```python
from build123d import *

# Parameters (mm, degrees)
F1_DEPTH = 38.1
F2_DEPTH = 63.5
F3_R     = 12.703802
F4_DEPTH = 65.251941


with BuildPart() as f1:
    # F0 (on Front) → F1 (new body, symmetric)
    with BuildSketch(Plane.XZ):
        with BuildLine():
            Line((-25.716836, 32.62547), (-67.867137, 32.62547))
            Line((-67.867137, 32.62547), (-67.867137, -32.62547))
            Line((-67.867137, -32.62547), (67.867137, -32.62547))
            Line((67.867137, -32.62547), (67.867137, 32.62547))
            Line((67.867137, 32.62547), (25.716836, 32.62547))
            ThreePointArc((25.716836, 32.62547), (0, 6.908634), (-25.716836, 32.62547))
        make_face()
    extrude(amount=F1_DEPTH, both=True)

    # F0 (on Front) → F2 (join, symmetric)
    with BuildSketch(Plane.XZ):
        with BuildLine():
            Line((-15.157554, 32.62547), (-25.716836, 32.62547))
            ThreePointArc((-25.716836, 32.62547), (0, 6.908634), (25.716836, 32.62547))
            Line((25.716836, 32.62547), (15.157554, 32.62547))
            ThreePointArc((15.157554, 32.62547), (0, 17.467917), (-15.157554, 32.62547))
        make_face()
    extrude(amount=F2_DEPTH, both=True)

    # F3 (on face) → F4 (cut, through all)
    with BuildSketch(Plane.XY.offset(32.62547)):
        with Locations((-43.029986, 0)):
            Circle(F3_R)
        with Locations((43.029986, 0)):
            Circle(F3_R)
    extrude(amount=-F4_DEPTH, mode=Mode.SUBTRACT)


solid = f1.part
```
Geometry check sheet. Reference: the model listing, model coordinates, mm. A direction names the side the tool comes from. Coordinates: 2 decimals unless noted, no trailing zeros. Write each loop counter-clockwise with the first axis right and the second up, starting at its lowest first coordinate (ties: lowest second). Pieces come first, ordered by that corner, then holes. Notation, with made-up numbers: (34.5, -22.5) -> (76.5, -22.5) arc R20 cw to (76.5, 2.5) -> close; hole circle Ø6 at (34.25, 51). An arc over 180 degrees is marked (long way). Use CSV: the item, a comma, the result in double quotes. Start each with the question number.
Item 1: Cross-section at D-D, the plane z = 14. Record the cut outline in (x, y).
Item 2: Mould release check, pull along X, two halves, no side actions. Record for faces 1 (the cylindrical face through (30.34, 0.56, 0.46)), 2 (the flat face through (-67.867, -1, 0)), 3 (the flat face through (0, 63.5, 17)), 4 (the flat face through (67.867, -1, 0)): released by +X, released by -X, zero draft, split by the parting line, or undercut.
Item 3: Cross-section at C-C, the plane y = 0. Record the cut outline in (x, z).
Item 4: Set-up check for faces 5 (the flat face through (30, -1, 32.625)), 6 (the cylindrical face through (-0.565, -50.978, 6.915)), 7 (the flat face through (-1, 38.1, 0)): record each of +Z, -Z, +X, -X, +Y, -Y from which the full face is reachable in a straight line by a thin tool's end or side.
Item 5: Cross-section at A-A, the plane z = 23.5. Record the cut outline in (x, y).
Item 6: Depth check by flat-ended pin: pin 1 Ø12 at (x, z) = (30.5, 22) entering from -Y; pin 2 Ø1.5 at (x, y) = (-7.5, 39.5) entering from -Z; pin 3 Ø1.5 at (x, y) = (24.5, 41.5) entering from -Z. Enter the tip coordinate at first touch or a pass-through.
Item 7: Thickness scan on line 1 (Y direction, x = -32, z = -2); line 2 (X direction, y = 46, z = 23); line 3 (Y direction, x = -62, z = -20). Record the ranges inside material, lowest first.
Item 8: Cross-section at B-B, the plane x = 40.5. Record the cut outline in (y, z).
Answers:
1,outline,"(-67.87, -38.1) -> (-17.73, -38.1) -> (-17.73, -63.5) -> (17.73, -63.5) -> (17.73, -38.1) -> (67.87, -38.1) -> (67.87, 38.1) -> (17.73, 38.1) -> (17.73, 63.5) -> (-17.73, 63.5) -> (-17.73, 38.1) -> (-67.87, 38.1) -> close; hole circle Ø25.41 at (-43.03, 0); hole circle Ø25.41 at (43.03, 0)"
2,face 1,"undercut"
2,face 2,"released by -X"
2,face 3,"zero draft"
2,face 4,"released by +X"
3,outline,"(-67.87, -32.63) -> (-55.73, -32.63) -> (-55.73, 32.63) -> (-67.87, 32.63) -> close; (-30.33, -32.63) -> (30.33, -32.63) -> (30.33, 32.63) -> (15.16, 32.63) arc R15.16 cw to (-15.16, 32.63) -> (-30.33, 32.63) -> close; (55.73, -32.63) -> (67.87, -32.63) -> (67.87, 32.63) -> (55.73, 32.63) -> close"
4,face 5,"+Z, +X, -X, +Y, -Y"
4,face 6,"-Z, -Y"
4,face 7,"-Z, +Y"
5,outline,"(-67.87, -38.1) -> (-24.04, -38.1) -> (-24.04, -63.5) -> (-12.1, -63.5) -> (-12.1, 63.5) -> (-24.04, 63.5) -> (-24.04, 38.1) -> (-67.87, 38.1) -> close; (12.1, -63.5) -> (24.04, -63.5) -> (24.04, -38.1) -> (67.87, -38.1) -> (67.87, 38.1) -> (24.04, 38.1) -> (24.04, 63.5) -> (12.1, 63.5) -> close; hole circle Ø25.41 at (-43.03, 0); hole circle Ø25.41 at (43.03, 0)"
6,pin 1,"y = -38.1"
6,pin 2,"z = 7.81"
6,pin 3,"z = 22.76"
7,line 1,"-38.1 to -6.3, 6.3 to 38.1"
7,line 2,"-23.85 to -11.71, 11.71 to 23.85"
7,line 3,"-38.1 to 38.1"
8,outline,"(-38.1, -32.63) -> (-12.45, -32.63) -> (-12.45, 32.63) -> (-38.1, 32.63) -> close; (12.45, -32.63) -> (38.1, -32.63) -> (38.1, 32.63) -> (12.45, 32.63) -> close"
